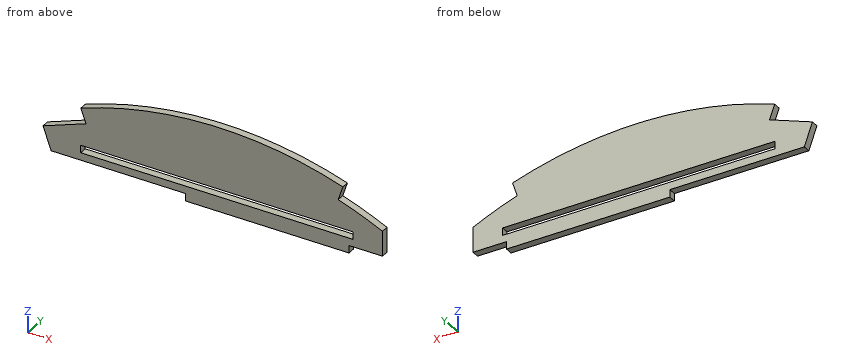
```python
from build123d import *

# Parameters (mm, degrees)
F0_W     = 400
F0_H     = 11
F1_DEPTH = 11


# Not quite as in the source:
# - ends of sketch curves that miss each other by under 0.0002 mm in the source are joined


with BuildPart() as f1:
    # F0 (on Front) → F1 (new body)
    with BuildSketch(Plane.XZ):
        with BuildLine():
            Line((-186.2102279461, 5.2641338535), (-249.389773, -18))
            Line((-249.389773, -18), (-237.378755, -51))
            Line((-237.378755, -51), (-39.805119, -51))
            Line((-39.805119, -51), (-39.805119, -62))
            Line((-39.805119, -62), (200.194881, -62))
            Line((200.194881, -62), (200.194881, -51))
            Line((200.194881, -51), (249.389772, -51))
            Line((249.389772, -51), (249.389772, -14.186388))
            ThreePointArc((249.389772, -14.186388), (217.2940285637, -0.1866284114), (184.3897718043, 11.7900114054))
            Line((184.3897718043, 11.7900114054), (191.267695, 32.687241))
            ThreePointArc((191.267695, 32.687241), (-1.7442805029, 61.9112120177), (-193.620736559, 25.9794888024))
            Line((-193.620736559, 25.9794888024), (-193.812138, 25.909012))
            Line((-193.812138, 25.909012), (-186.2102279461, 5.2641338535))
        make_face()
        with Locations((6.005508, -34.5)):
            Rectangle(F0_W, F0_H, mode=Mode.SUBTRACT)
    extrude(amount=F1_DEPTH)


solid = f1.part
```
Can you work these out from the model? Positions are in its coordinate system, mm. Give positions to 0.01 mm unless a question says otherwise; leave off trailing zeros. Write each loop counter-clockwise with the first axis right and the second up, starting at its lowest first coordinate (ties: lowest second). Pieces come first, ordered by that corner, then holes. Notation, with made-up numbers: (69, 10.5) -> (97, 10.5) arc R14 cw to (97, 33.5) -> close; hole circle Ø3 at (81, 6.5). An arc over 180 degrees is marked (long way). One line per item, written item: value.
Q1. Imagine slicing it at A-A on y = -6.5. Please give me the cut outline in (x, z).
Results found:
outline: (-249.39, -18) -> (-237.38, -51) -> (-39.81, -51) -> (-39.81, -62) -> (200.19, -62) -> (200.19, -51) -> (249.39, -51) -> (249.39, -14.19) arc R562.78 ccw to (184.39, 11.79) -> (191.27, 32.69) arc R584.78 ccw to (-193.62, 25.98) -> (-193.81, 25.91) -> (-186.21, 5.26) -> close; hole (-193.99, -40) -> (206.01, -40) -> (206.01, -29) -> (-193.99, -29) -> close
Q2. For P1, Ø4, axis at y = -7, z = 28, coming from the +X side; P2, Ø5, axis at y = -7, z = -48, coming from the -X side; P3, Ø6, axis at x = 144.5, y = -4, coming from the +Z side, each with a flat end and sliding along its axis, tell me the tip position at first contact or that it passes through.
Results found:
P1: stops at x = 190.38
P2: stops at x = -239.38
P3: stops at z = 46.66
Q3. Imagine slicing it at B-B on x = 178. Please give me the cut outline in (y, z).
Results found:
outline: (-11, -62) -> (0, -62) -> (0, -40) -> (-11, -40) -> close; (-11, -29) -> (0, -29) -> (0, 36.88) -> (-11, 36.88) -> close
Q4. Please list where these lines run through material, in increasing order: line 1 (Z direction, x = -17.5, y = -4.25); line 2 (Z direction, x = -185.5, y = -2); line 3 (X direction, y = -4.25, z = -30.5). Write a range as [from, to].
Results found:
line 1: z = [-62, -40], [-29, 61.42]
line 2: z = [-51, -40], [-29, 28.9]
line 3: x = [-244.84, -193.99], [206.01, 249.39]
Q5. Imagine slicing it at C-C on x = -31. Please give me the cut outline in (y, z), and give its area (3 significant figures).
Results found:
outline: (-11, -62) -> (0, -62) -> (0, -40) -> (-11, -40) -> close; (-11, -29) -> (0, -29) -> (0, 60.67) -> (-11, 60.67) -> close
area: 1,230 mm^2
Q6. Imagine slicing it at D-D on z = -10. Please give me the cut outline in (x, y), and give its area (3 significant figures).
Results found:
outline: (-227.66, -11) -> (240.35, -11) -> (240.35, 0) -> (-227.66, 0) -> close
area: 5,150 mm^2
